Source: CAD feature listing. Evaluate the final solid. Frame: model axes, mm. A direction names the side the tool comes from. Round coordinates to 2 decimals unless told otherwise and drop trailing zeros. Order: outer loops, then holes, each group sorted by start corner. A loop starts at its lowest first (then second) coordinate and runs counter-clockwise, first axis right, second up. Notation, with made-up numbers: (22.25, 15) - (28.25, 15) arc R8 ccw to (28.25, 22) - close; hole circle Ø3 at (76, -20). An arc over 180 degrees is marked (long way). Put each result on its own line as item: value. Start each with the question number.
1) Access query for faces 4 (the face through (24.45, -1.01, 12.08)), 5 (the face through (-22.645, -0.514, 10.896)), 6 (the face through (26.45, 0.49, -12.04)), 7 (the face through (0, 0.5, 0)), 8 (the face through (-23.5, 1, 0)). Directions: +Z, -Z, +X, -X, +Y, -Y. A direction counts if a zero-diameter tool reaches every point of the face in a straight line with its end or side. Return the directions, or none.
2) Section B-B on z = 12. Output: boundary loops of the cut face in (x, y).
3) Contact query for flat-ended pins moving along their axis: P1, Ø8, axis at x = 37, z = -13.5, coming from the -Y side; P2, Ø0.8, axis at x = 34, y = -1, coming from the +Z side; P3, Ø2, axis at x = 31, z = 12, coming from the -Y side; P4, Ø5, axis at x = -7.5, z = -8.5, coming from the +Y side. Output: stop coordinate, or through.
4) Mould query, pull axis Z, two halves, no side actions, for faces 1 (the face through (1, -1.5, 0)), 2 (the face through (0, 0, 9.994)), 3 (the face through (-42.55, -1.01, -11.92)). Classes: +Z half, -Z half, draft (parallel to the pull), parting line (faces both ways), or undercut.
5) Section C-C on z = 1.5. Output: boundary loops of the cut face in (x, y), then the cut area to 3 significant figures.
6) Line query: probe 1 along X at (y, z) = (0.65, -15); probe 2 along Z at (x, y) = (26, -0.6); probe 3 along Z at (x, y) = (-28, 1). Output: solid intervals per line, ascending. Write a range as [from, to].
7) Section A-A on x = 31.5. Output: boundary loops of the cut face in (y, z), then the cut area to 3 significant figures.
8) Section D-D on x = -16.5. Output: boundary loops of the cut face in (y, z).
```python
from build123d import *

# Parameters (mm, degrees)
EXTRUDE_1_DEPTH     = 43.5
SKETCH_3_W          = 47
SKETCH_3_H          = 40
CUT_EXTRUDE_1_DEPTH = 1
SKETCH_4_W          = 47
SKETCH_4_H          = 16.028408988
CUT_EXTRUDE_2_DEPTH = 48.919202831
CUT_EXTRUDE_3_DEPTH = 48.971345614
CUT_EXTRUDE_4_DEPTH = 1
FILLET_1_R          = 3


with BuildPart() as part:
    # 草图2 → 凸台-拉伸1 (new, symmetric)
    with BuildSketch(Plane(origin=(0, 0, 0), x_dir=(0, 0, -1), z_dir=(1, 0, 0))):
        with BuildLine():
            Line((-18.5, 1.5), (18.5, 1.5))
            ThreePointArc((18.5, 1.5), (20, 0), (18.5, -1.5))
            Line((18.5, -1.5), (-18.5, -1.5))
            ThreePointArc((-18.5, -1.5), (-20, 0), (-18.5, 1.5))
        make_face()
    extrude(amount=EXTRUDE_1_DEPTH, both=True)

    # 草图3 → 切除-拉伸1 (cut)
    with BuildSketch(Plane(origin=(0, 1.5, 0), x_dir=(1, 0, 0), z_dir=(0, 1, 0))):
        Rectangle(SKETCH_3_W, SKETCH_3_H)
    extrude(amount=-CUT_EXTRUDE_1_DEPTH, mode=Mode.SUBTRACT)

    # 草图4 → 切除-拉伸2 (cut, through all)
    with BuildSketch(Plane(origin=(0, 0.5, 0), x_dir=(1, 0, 0), z_dir=(0, 1, 0))):
        with Locations((0, 18.008457368)):
            Rectangle(SKETCH_4_W, SKETCH_4_H)
        with Locations((0, -18.008457368)):
            Rectangle(SKETCH_4_W, SKETCH_4_H)
    extrude(amount=-CUT_EXTRUDE_2_DEPTH, mode=Mode.SUBTRACT)

    # 草图5 → 切除-拉伸3 (cut, through all)
    with BuildSketch(Plane(origin=(0, -1.5, 0), x_dir=(-1, 0, 0), z_dir=(0, -1, 0))):
        with BuildLine():
            Line((38.8, -13.75), (28.2, -13.75))
            ThreePointArc((28.2, -13.75), (26.45, -12), (28.2, -10.25))
            Line((28.2, -10.25), (38.8, -10.25))
            ThreePointArc((38.8, -10.25), (40.55, -12), (38.8, -13.75))
        make_face()
        with BuildLine():
            Line((38.8, 13.75), (28.2, 13.75))
            ThreePointArc((28.2, 13.75), (26.45, 12), (28.2, 10.25))
            Line((28.2, 10.25), (38.8, 10.25))
            ThreePointArc((38.8, 10.25), (40.55, 12), (38.8, 13.75))
        make_face()
        with BuildLine():
            Line((-38.8, 13.75), (-28.2, 13.75))
            ThreePointArc((-28.2, 13.75), (-26.45, 12), (-28.2, 10.25))
            Line((-28.2, 10.25), (-38.8, 10.25))
            ThreePointArc((-38.8, 10.25), (-40.55, 12), (-38.8, 13.75))
        make_face()
        with BuildLine():
            Line((-38.8, -13.75), (-28.2, -13.75))
            ThreePointArc((-28.2, -13.75), (-26.45, -12), (-28.2, -10.25))
            Line((-28.2, -10.25), (-38.8, -10.25))
            ThreePointArc((-38.8, -10.25), (-40.55, -12), (-38.8, -13.75))
        make_face()
    extrude(amount=-CUT_EXTRUDE_3_DEPTH, mode=Mode.SUBTRACT)

    # 草图6 → 切除-拉伸4 (cut)
    with BuildSketch(Plane.XZ.offset(1.5)):
        with BuildLine():
            Line((-28.2, 15.75), (-38.8, 15.75))
            ThreePointArc((-38.8, 15.75), (-42.55, 12), (-38.8, 8.25))
            Line((-38.8, 8.25), (-28.2, 8.25))
            ThreePointArc((-28.2, 8.25), (-24.45, 12), (-28.2, 15.75))
        make_face()
        with BuildLine():
            Line((-38.8, -15.75), (-28.2, -15.75))
            ThreePointArc((-28.2, -15.75), (-24.45, -12), (-28.2, -8.25))
            Line((-28.2, -8.25), (-38.8, -8.25))
            ThreePointArc((-38.8, -8.25), (-42.55, -12), (-38.8, -15.75))
        make_face()
        with BuildLine():
            Line((38.8, 15.75), (28.2, 15.75))
            ThreePointArc((28.2, 15.75), (24.45, 12), (28.2, 8.25))
            Line((28.2, 8.25), (38.8, 8.25))
            ThreePointArc((38.8, 8.25), (42.55, 12), (38.8, 15.75))
        make_face()
        with BuildLine():
            Line((28.2, -15.75), (38.8, -15.75))
            ThreePointArc((38.8, -15.75), (42.55, -12), (38.8, -8.25))
            Line((38.8, -8.25), (28.2, -8.25))
            ThreePointArc((28.2, -8.25), (24.45, -12), (28.2, -15.75))
        make_face()
    extrude(amount=-CUT_EXTRUDE_4_DEPTH, mode=Mode.SUBTRACT)

    # 圆角1
    fillet_1_edges = [part.edges().sort_by_distance(p)[0] for p in [
        (-23.5, -0.5, -9.994252874),
        (23.5, -0.5, -9.994252874),
        (23.5, -0.5, 9.994252874),
        (-23.5, -0.5, 9.994252874),
    ]]
    fillet(fillet_1_edges, radius=FILLET_1_R)


solid = part.part
```
Answer sheet:
1. face 4: -Y
1. face 5: +Z, +Y, -Y
1. face 6: +Y, -Y
1. face 7: +Z, -Z, +Y
1. face 8: +Y
2. outline: (-43.5, -1.5) - (-42.55, -1.5) - (-42.55, -0.5) - (-40.55, -0.5) - (-40.55, 1.5) - (-43.5, 1.5) - close; (-26.45, -0.5) - (-24.45, -0.5) - (-24.45, -1.5) - (-23.33, -1.5) - (-23.33, 0.5) - (-23.5, 0.5) - (-23.5, 1.5) - (-26.45, 1.5) - close; (23.33, -1.5) - (24.45, -1.5) - (24.45, -0.5) - (26.45, -0.5) - (26.45, 1.5) - (23.5, 1.5) - (23.5, 0.5) - (23.33, 0.5) - close; (40.55, -0.5) - (42.55, -0.5) - (42.55, -1.5) - (43.5, -1.5) - (43.5, 1.5) - (40.55, 1.5) - close
3. P1: y = -1.5
3. P2: z = 19.87
3. P3: through
3. P4: y = 0.5
4. face 1: draft
4. face 2: +Z half
4. face 3: undercut
5. outline: (-43.5, -1.5) - (43.5, -1.5) - (43.5, 1.5) - (23.5, 1.5) - (23.5, 0.5) - (-23.5, 0.5) - (-23.5, 1.5) - (-43.5, 1.5) - close
5. area: 214 mm^2
6. probe 1: [-43.5, -23.5], [23.5, 43.5]
6. probe 2: [-19.87, -15.04], [-8.96, 8.96], [15.04, 19.87]
6. probe 3: [-19.62, -13.74], [-10.26, 10.26], [13.74, 19.62]
7. outline: (-1.5, -18.5) arc R1.5 ccw to (1.5, -18.5) - (1.5, -13.75) - (-0.5, -13.75) - (-0.5, -15.75) - (-1.5, -15.75) - close; (-1.5, -8.25) - (-0.5, -8.25) - (-0.5, -10.25) - (1.5, -10.25) - (1.5, 10.25) - (-0.5, 10.25) - (-0.5, 8.25) - (-1.5, 8.25) - close; (-1.5, 15.75) - (-0.5, 15.75) - (-0.5, 13.75) - (1.5, 13.75) - (1.5, 18.5) arc R1.5 ccw to (-1.5, 18.5) - close
7. area: 89.1 mm^2
8. outline: (-1.5, -9.99) - (0.5, -9.99) - (0.5, 9.99) - (-1.5, 9.99) - close
